Here's how the part is built. I have some questions about the finished solid (model axes, mm). A direction names the side the tool comes from. Give positions to 0.01 mm unless a question says otherwise; leave off trailing zeros. Loops run counter-clockwise (first coordinate to the right, second up) from the corner with the lowest first, then second, coordinate; pieces in that order, holes last. Notation, with made-up numbers: (-9.75, -30.75) - (25.25, -30.75) arc R19 cw to (25.25, -24.75) - close; hole circle Ø11 at (66.5, 71). An arc over 180 degrees is marked (long way). Use a Markdown table: item, result.
from build123d import *

# Parameters (mm, degrees)
SKETCH_5_R          = 6.5
EXTRUDE_5_DEPTH     = 1.3
SKETCH_6_R          = 5.85
EXTRUDE_6_DEPTH     = 4.4
FILLET_2_R          = 0.5
SKETCH_7_W          = 4
SKETCH_7_H          = 4
EXTRUDE_7_DEPTH     = 2
SKETCH_8_W          = 3.8
SKETCH_8_H          = 3.8
CUT_EXTRUDE_1_DEPTH = 2


with BuildPart() as part:
    # Эскиз5 → Бобышка-Вытянуть5 (new body)
    with BuildSketch(Plane(origin=(0, 0, 0), x_dir=(1, 0, 0), z_dir=(0, 1, 0))):
        Circle(SKETCH_5_R)
    extrude(amount=EXTRUDE_5_DEPTH)

    # Эскиз6 → Бобышка-Вытянуть6 (add)
    with BuildSketch(Plane(origin=(0, 1.3, 0), x_dir=(1, 0, 0), z_dir=(0, 1, 0))):
        Circle(SKETCH_6_R)
    extrude(amount=EXTRUDE_6_DEPTH)

    # Скругление2
    fillet_2_edges = [part.edges().sort_by_distance(p)[0] for p in [
        (-5.85, 5.7, 0),
    ]]
    fillet(fillet_2_edges, radius=FILLET_2_R)

    # Эскиз7 → Бобышка-Вытянуть7 (add)
    with BuildSketch(Plane.XZ):
        Rectangle(SKETCH_7_W, SKETCH_7_H)
    extrude(amount=EXTRUDE_7_DEPTH)

    # Эскиз8 → Вырез-Вытянуть1 (cut)
    with BuildSketch(Plane.XZ.offset(2)):
        Rectangle(SKETCH_8_W, SKETCH_8_H)
    extrude(amount=-CUT_EXTRUDE_1_DEPTH, mode=Mode.SUBTRACT)


solid = part.part
(1) Suppose I cut it at B-B on x = 0. Write out the boundary of the cut face in (y, z), plus the area to 3 significant figures.
A:
| item | result |
|---|---|
| outline | (-2, -2) - (0, -2) - (0, -6.5) - (1.3, -6.5) - (1.3, -5.85) - (5.2, -5.85) arc R0.5 ccw to (5.7, -5.35) - (5.7, 5.35) arc R0.5 ccw to (5.2, 5.85) - (1.3, 5.85) - (1.3, 6.5) - (0, 6.5) - (0, 2) - (-2, 2) - (-2, 1.9) - (0, 1.9) - (0, -1.9) - (-2, -1.9) - close |
| area | 68.7 mm2 |
(2) If I drill on line 1 (Y direction, x = 4.5, z = 1.25); line 2 (Y direction, x = -3.75, z = -4.75); line 3 (Z direction, x = -4.75, y = 1), over which ranges is the centre line in solid material (lowest first)?
A:
| item | result |
|---|---|
| line 1 | 0 to 5.7 |
| line 2 | 0 to 1.3 |
| line 3 | -4.44 to 4.44 |
(3) Suppose I cut it at A-A on z = 0. Write out the boundary of the cut face in (x, y).
A:
| item | result |
|---|---|
| outline | (-6.5, 0) - (-2, 0) - (-2, -2) - (-1.9, -2) - (-1.9, 0) - (1.9, 0) - (1.9, -2) - (2, -2) - (2, 0) - (6.5, 0) - (6.5, 1.3) - (5.85, 1.3) - (5.85, 5.2) arc R0.5 ccw to (5.35, 5.7) - (-5.35, 5.7) arc R0.5 ccw to (-5.85, 5.2) - (-5.85, 1.3) - (-6.5, 1.3) - close |
(4) Suppose I cut it at C-C on y = 4.25. Write out the boundary of the cut face in (x, z), plus the area to 3 significant figures.
A:
| item | result |
|---|---|
| outline | circle Ø11.7 at (0, 0) |
| area | 108 mm2 |
(5) We'd pull the mould along Z, two halves only. Please class faces 3 (the face through (-5.158, 0.641, 3.955)), 4 (the face through (3, 0, 0)), 5 (the face through (0, 0, 0)): pulls with the +Z half, pulls with the -Z half, needs draft (parallel to the pull), parting line crosses it, or undercut.
A:
| item | result |
|---|---|
| face 3 | parting line crosses it |
| face 4 | needs draft |
| face 5 | undercut |
(6) Will these pins go through, and if not, where does the flat tip stop? pin 1 (4 mm diameter, centred on x = 4, y = -0.5, fed in from +Z); pin 2 (1.6 mm diameter, centred on x = 1, y = -1, fed in from -Z); pin 3 (1.9 mm diameter, centred on x = 0.5, z = 0, fed in from -Y).
A:
| item | result |
|---|---|
| pin 1 | z = 6.16 |
| pin 2 | z = -2 |
| pin 3 | y = 0 |
(7) On a 3-axis mill with a long thin cutter (end or side, diameter ignored), from which of +Z, -Z, +X, -X, +Y, -Y can I reach the whole of each face in a straight line? I mean faces 1 (the face through (-1.27, 3.22, 5.71)), 2 (the face through (0, 5.7, 0)). Say none if no direction works.
A:
| item | result |
|---|---|
| face 1 | +Y |
| face 2 | +Z, -Z, +X, -X, +Y |
